The listing builds one solid part. Answer for the finished solid, in the listing's coordinates (mm). Round coordinates to 2 decimals unless told otherwise and drop trailing zeros. Order: outer loops, then holes, each group sorted by start corner. A loop starts at its lowest first (then second) coordinate and runs counter-clockwise, first axis right, second up. Notation, with made-up numbers: (52, 77.25) - (103, 77.25) arc R21 cw to (103, 90.25) - close; hole circle Ø11 at (-17.5, 85). An arc over 180 degrees is marked (long way). One line per item, written item: value. Start each with the question number.
1. Section B-B, the plane z = 17 is taken. Give the vertices of the cut face in (x, y).
2. Straight lines are drawn through the part: line 1 (X direction, y = 50.5, z = 18); line 2 (Y direction, x = -5, z = 5); line 3 (Y direction, x = 5.5, z = 4.5). For each, find the intervals that lie inside material, in ascending order.
3. Section A-A, the plane y = 42 is taken. Give the vertices of the cut face in (x, z).
from build123d import *

# Parameters (mm, degrees)
PAD006_DEPTH               = 21
PAD006_MIRRORED002_2_DEPTH = 21


with BuildPart() as part:
    # Sketch006 → Pad006 (new body)
    with BuildSketch(Plane.XY):
        with BuildLine():
            Line((0, 0), (19, 0))
            Line((19, 0), (19, 63.5))
            Line((19, 63.5), (0, 63.5))
            Line((0, 63.5), (0, 57))
            ThreePointArc((6.5, 50.5), (4.596194, 55.096194), (0, 57))
            Line((6.5, 44.5), (6.5, 50.5))
            ThreePointArc((-0.001235, 38), (4.595757, 39.903369), (6.5, 44.5))
            Line((-0.001235, 38), (0, 0))
        make_face()
    pad006 = extrude(amount=PAD006_DEPTH)

    # Sketch006 Mirrored002 2 → Pad006 Mirrored002 2 (add)
    with BuildSketch(Plane(origin=(0, 0, 0), x_dir=(-1, 0, 0), z_dir=(0, 0, -1))):
        with BuildLine():
            Line((0, 0), (19, 0))
            Line((19, 0), (19, 63.5))
            Line((19, 63.5), (0, 63.5))
            Line((0, 63.5), (0, 57))
            ThreePointArc((6.5, 50.5), (4.596194, 55.096194), (0, 57))
            Line((6.5, 44.5), (6.5, 50.5))
            ThreePointArc((-0.001235, 38), (4.595757, 39.903369), (6.5, 44.5))
            Line((-0.001235, 38), (0, 0))
        make_face()
    pad006_mirrored002_2 = extrude(amount=-PAD006_MIRRORED002_2_DEPTH)

    # Mirrored003: Pad006, Pad006 Mirrored002 2 across Sketch006 H_Axis
    add(pad006.mirror(Plane.ZX))
    add(pad006_mirrored002_2.mirror(Plane.ZX))


solid = part.part
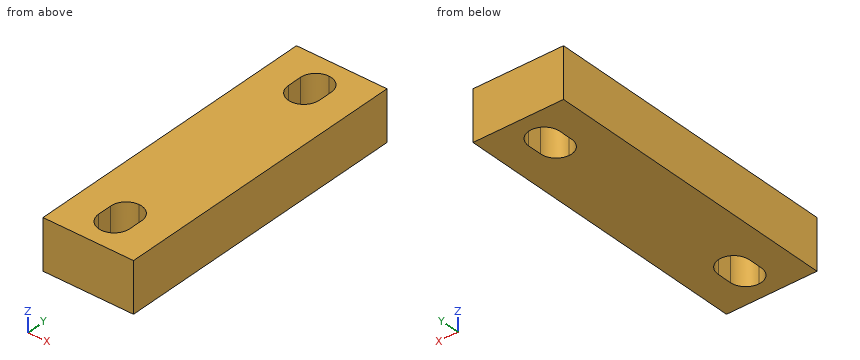
Answer list:
1. outline: (-19, -63.5) - (19, -63.5) - (19, 63.5) - (-19, 63.5) - close; hole (-6.5, -50.5) arc R6.5 ccw to (6.5, -50.5) - (6.5, -44.5) arc R6.5 ccw to (-6.5, -44.5) - close; hole (-6.5, 44.5) arc R6.5 ccw to (6.5, 44.5) - (6.5, 50.5) arc R6.5 ccw to (-6.5, 50.5) - close
2. line 1: x = -19 to -6.5, 6.5 to 19
2. line 2: y = -63.5 to -54.65, -40.35 to 40.35, 54.65 to 63.5
2. line 3: y = -63.5 to -53.96, -41.04 to 41.04, 53.96 to 63.5
3. outline: (-19, 0) - (-6, 0) - (-6, 21) - (-19, 21) - close; (6, 0) - (19, 0) - (19, 21) - (6, 21) - close
